```python
from build123d import *

# Parameters (mm, degrees)
SKETCH_W            = 219
SKETCH_H            = 134
PAD_DEPTH           = 2
SKETCH001_R         = 5
SKETCH001_R_2       = 2.75
POCKET_DEPTH        = 2.001
LINEARPATTERN_COUNT = 6
LINEARPATTERN_PITCH = 34
SKETCH002_W         = 219
SKETCH002_H         = 1
POCKET001_DEPTH     = 1


with BuildPart() as part:
    # Sketch (on Sketch) → Pad (new body)
    with BuildSketch(Plane.XY):
        Rectangle(SKETCH_W, SKETCH_H)
    extrude(amount=PAD_DEPTH)

    # Sketch001 → Pocket (cut, through all)
    with BuildSketch(Plane.XY):
        with Locations((-95.5, 39)):
            Circle(SKETCH001_R)
        with Locations((-95.5, 13)):
            Circle(SKETCH001_R)
        with Locations((-95.5, -13)):
            Circle(SKETCH001_R)
        with Locations((-95.5, -39)):
            Circle(SKETCH001_R)
        with Locations((-79.5, 39)):
            Circle(SKETCH001_R_2)
        with Locations((-79.5, 13)):
            Circle(SKETCH001_R_2)
        with Locations((-79.5, -13)):
            Circle(SKETCH001_R_2)
        with Locations((-79.5, -39)):
            Circle(SKETCH001_R_2)
    pocket = extrude(amount=POCKET_DEPTH, mode=Mode.SUBTRACT)

    # LinearPattern: Pocket ×6
    with Locations(*[(i * LINEARPATTERN_PITCH, 0, 0) for i in range(1, LINEARPATTERN_COUNT)]):
        add(pocket, mode=Mode.SUBTRACT)

    # Sketch002 (on Face5 of LinearPattern) → Pocket001 (cut)
    with BuildSketch(Plane.XY.offset(2)):
        with Locations((0, 66.5)):
            Rectangle(SKETCH002_W, SKETCH002_H)
    pocket001 = extrude(amount=-POCKET001_DEPTH, mode=Mode.SUBTRACT)

    # Mirrored: Pocket001 across XZ
    add(pocket001.mirror(Plane.XZ), mode=Mode.SUBTRACT)


solid = part.part
```
CAD build for the part. Positions are in the model's coordinates, mm. Give positions to 0.01 mm unless a question says otherwise; leave off trailing zeros. Loops run counter-clockwise (first coordinate to the right, second up) from the corner with the lowest first, then second, coordinate; pieces in that order, holes last. Notation, with made-up numbers: (24.5, 51) - (72.5, 51) arc R17 cw to (72.5, 84) - close; hole circle Ø6 at (53, 56.5). An arc over 180 degrees is marked (long way). Put each result on its own line as item: value.
Q1. Probe line 1 along Y through (x, z) = (22.5, 0.75); line 2 along Y through (x, z) = (10.5, 1.45); line 3 along Y through (x, z) = (-17, 1.25). List the from-to ranges inside material, lowest first.
Filled in:
line 1: y = -67 to -41.75, -36.25 to -15.75, -10.25 to 10.25, 15.75 to 36.25, 41.75 to 67
line 2: y = -66 to -42, -36 to -16, -10 to 10, 16 to 36, 42 to 66
line 3: y = -66 to 66
Q2. Slice it at C-C (x = 40.5). Give the cut face in (y, z), plus the area to 3 significant figures.
Filled in:
outline: (-67, 0) - (-44, 0) - (-44, 2) - (-66, 2) - (-66, 1) - (-67, 1) - close; (-34, 0) - (-18, 0) - (-18, 2) - (-34, 2) - close; (-8, 0) - (8, 0) - (8, 2) - (-8, 2) - close; (18, 0) - (34, 0) - (34, 2) - (18, 2) - close; (44, 0) - (67, 0) - (67, 1) - (66, 1) - (66, 2) - (44, 2) - close
area: 186 mm²
Q3. Slice it at A-A (x = 90.5). Give the cut face in (y, z).
Filled in:
outline: (-67, 0) - (-41.75, 0) - (-41.75, 2) - (-66, 2) - (-66, 1) - (-67, 1) - close; (-36.25, 0) - (-15.75, 0) - (-15.75, 2) - (-36.25, 2) - close; (-10.25, 0) - (10.25, 0) - (10.25, 2) - (-10.25, 2) - close; (15.75, 0) - (36.25, 0) - (36.25, 2) - (15.75, 2) - close; (41.75, 0) - (67, 0) - (67, 1) - (66, 1) - (66, 2) - (41.75, 2) - close
Q4. Slice it at B-B (y = -13). Give the number of separate pieces and of enclosed holes in the cut face, plus the area to 3 significant figures.
Filled in:
separate pieces: 13
enclosed holes: 0
area: 252 mm²
Q5. Mould opens along Y. For faces 1 (the face through (-2, 1, 0)), 2 (the face through (87.753, -38.879, 0.986)) say: pulls with the +Y half, pulls with the -Y half, needs draft (parallel to the pull), parting line crosses it, or undercut.
Filled in:
face 1: needs draft
face 2: undercut
Q6. Flat gauge pin, fed straight in: pin 1 (11.5 mm diameter, centred on x = -61.5, y = -39, fed in from +Z). Where does the tip first touch, or does it go through?
Filled in:
pin 1: stops at z = 2
